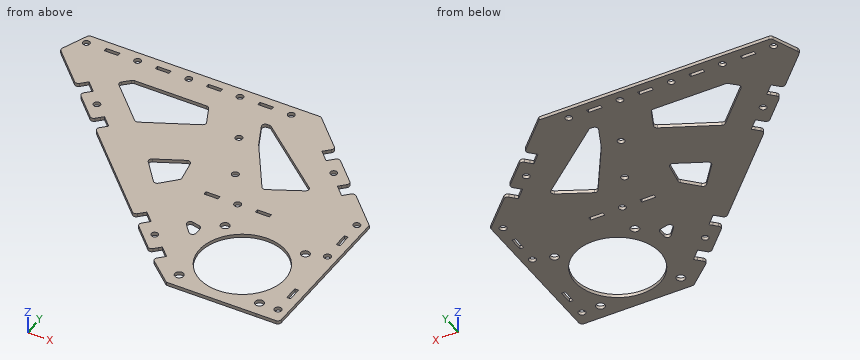
from build123d import *

# Parameters (mm, degrees)
SKETCH_1_R      = 2
SKETCH_1_R_2    = 25
SKETCH_1_R_3    = 2.05
SKETCH_1_R_4    = 2.55
SKETCH_1_W      = 8.1
SKETCH_1_H      = 2.1
SKETCH_1_W_2    = 8.2
SKETCH_1_W_3    = 2.2
SKETCH_1_H_2    = 8.2
EXTRUDE_1_DEPTH = 2
FILLET_2_R      = 2


with BuildPart() as part:
    # 草图1 → 凸台-拉伸1 (new body)
    with BuildSketch(Plane.XY):
        Polygon((7.027428163, -4.999036262), (20.810808237, -16.956988843), (73.227648339, -16.964389058), (87.027428163, -16.964389058), (87.027428163, 75.054738201), (67.497807203, 94.584359161), (63.997628636, 91.084180595), (62.512704395, 89.599256354), (56.785139468, 95.326821282), (58.270063708, 96.811745522), (61.771734574, 100.31043179), (54.027428163, 108.054738201), (46.284614051, 115.797552313), (42.784435485, 112.297373746), (41.299511244, 110.812449505), (35.571946316, 116.540014433), (37.056870557, 118.024938674), (40.557049124, 121.52511724), (21.027428163, 141.054738201), (-114.884210676, 141.054738201), (-121.955278488, 123.983670389), (-100.755816342, 102.784208243), (-97.257364322, 106.282660262), (-95.772440082, 107.767584503), (-90.044875154, 102.040019575), (-91.529799395, 100.555095335), (-95.028251414, 97.056643315), (-87.28543216, 89.313824061), (-79.542612906, 81.571004807), (-76.044160887, 85.069456827), (-74.559236646, 86.554381067), (-68.831671719, 80.82681614), (-70.316595959, 79.341891899), (-73.815047978, 75.84343988), (-21.559856849, 23.58824875), (-18.061404829, 27.086700769), (-16.576480589, 28.57162501), (-10.848915661, 22.844060082), (-12.333839902, 21.359135842), (-15.832291921, 17.860683822), (-8.089472667, 10.117864568), (-0.346653413, 2.375045314), (3.151798606, 5.873497334), (4.636722847, 7.358421574), (10.364287774, 1.630856647), (8.879363534, 0.145932406), (5.380911515, -3.352519613), align=None)
        with Locations((-52.972571837, 135.054738201)):
            Circle(SKETCH_1_R, mode=Mode.SUBTRACT)
        with Locations((47.027428163, 15.054738201)):
            Circle(SKETCH_1_R_2, mode=Mode.SUBTRACT)
        with Locations(Location((-22.972571837, 135.054738201, 0), (0, 0, 180))):
            Circle(SKETCH_1_R, mode=Mode.SUBTRACT)
        with Locations((7.027428163, 135.054738201)):
            Circle(SKETCH_1_R, mode=Mode.SUBTRACT)
        with Locations(Location((-112.972571837, 135.054738201, 0), (0, 0, 180))):
            Circle(SKETCH_1_R, mode=Mode.SUBTRACT)
        with Locations((-82.972571837, 135.054738201)):
            Circle(SKETCH_1_R, mode=Mode.SUBTRACT)
        with Locations((49.784787476, 103.812097514)):
            Circle(SKETCH_1_R, mode=Mode.SUBTRACT)
        with Locations((-83.04451802, 93.554738201)):
            Circle(SKETCH_1_R, mode=Mode.SUBTRACT)
        with Locations((20.275835807, 57.054738201)):
            Circle(SKETCH_1_R_3, mode=Mode.SUBTRACT)
        with Locations((70.527428163, -8.445261799)):
            Circle(SKETCH_1_R_4, mode=Mode.SUBTRACT)
        with Locations((23.527428163, -8.445261799)):
            Circle(SKETCH_1_R_4, mode=Mode.SUBTRACT)
        with Locations((23.527428163, 38.554738201)):
            Circle(SKETCH_1_R_4, mode=Mode.SUBTRACT)
        with Locations((70.527428163, 38.554738201)):
            Circle(SKETCH_1_R_4, mode=Mode.SUBTRACT)
        with Locations((81.392055944, 72.204829046)):
            Circle(SKETCH_1_R_3, mode=Mode.SUBTRACT)
        with Locations((81.392055944, -8.445261799)):
            Circle(SKETCH_1_R_3, mode=Mode.SUBTRACT)
        with Locations((81.392055944, 42.204829046)):
            Circle(SKETCH_1_R_3, mode=Mode.SUBTRACT)
        with Locations((6.845259268, 78.140743367)):
            Circle(SKETCH_1_R_3, mode=Mode.SUBTRACT)
        with Locations(Location((-3.848558527, 14.358778708, 0), (0, 0, 180))):
            Circle(SKETCH_1_R, mode=Mode.SUBTRACT)
        with Locations((-6.58531727, 105.226748532)):
            Circle(SKETCH_1_R_3, mode=Mode.SUBTRACT)
        with Locations((-37.972571837, 135.054738201)):
            Rectangle(SKETCH_1_W, SKETCH_1_H, mode=Mode.SUBTRACT)
        with Locations((-7.972571837, 135.054738201)):
            Rectangle(SKETCH_1_W, SKETCH_1_H, mode=Mode.SUBTRACT)
        with Locations((-97.972571837, 135.054738201)):
            Rectangle(SKETCH_1_W, SKETCH_1_H, mode=Mode.SUBTRACT)
        with Locations((-67.972571837, 135.054738201)):
            Rectangle(SKETCH_1_W, SKETCH_1_H, mode=Mode.SUBTRACT)
        with Locations((5.275835807, 57.054738201)):
            Rectangle(SKETCH_1_W_2, SKETCH_1_H, mode=Mode.SUBTRACT)
        with Locations((35.275835807, 57.054738201)):
            Rectangle(SKETCH_1_W_2, SKETCH_1_H, mode=Mode.SUBTRACT)
        Polygon((-26.317798475, 106.3059132), (-58.783300448, 90.506724064), (-82.786741677, 114.510165293), (-76.96930946, 120.054738201), (-32.606331473, 120.054738201), align=None, mode=Mode.SUBTRACT)
        Polygon((47.299709176, 85.219712632), (24.92619293, 73.952191934), (4.862626833, 105.451990707), (-2.731253041, 122.054738201), (2.37892986, 122.054738201), align=None, mode=Mode.SUBTRACT)
        Polygon((-14.950211349, 60.939664471), (-17.845757969, 77.065019133), (-38.30861977, 67.106860342), (-24.982934729, 50.626518371), align=None, mode=Mode.SUBTRACT)
        Polygon((2.01437662, 34.262984309), (13.802642778, 20.368597473), (13.802642778, 31.594822975), align=None, mode=Mode.SUBTRACT)
        with Locations((81.392055944, 57.204829046)):
            Rectangle(SKETCH_1_W_3, SKETCH_1_H_2, mode=Mode.SUBTRACT)
        with Locations((81.392055944, 6.554738201)):
            Rectangle(SKETCH_1_W_3, SKETCH_1_H_2, mode=Mode.SUBTRACT)
    extrude(amount=EXTRUDE_1_DEPTH)

    # 圆角2
    fillet_2_edges = [part.edges().sort_by_distance(p)[0] for p in [
        (-26.317798475, 106.3059132, 1),
        (-32.606331473, 120.054738201, 1),
        (-76.96930946, 120.054738201, 1),
        (-82.786741677, 114.510165293, 1),
        (-58.783300448, 90.506724064, 1),
        (47.299709176, 85.219712632, 1),
        (2.37892986, 122.054738201, 1),
        (-2.731253041, 122.054738201, 1),
        (24.92619293, 73.952191934, 1),
        (-24.982934729, 50.626518371, 1),
        (-14.950211349, 60.939664471, 1),
        (-17.845757969, 77.065019133, 1),
        (-38.30861977, 67.106860342, 1),
        (13.802642778, 31.594822975, 1),
        (2.01437662, 34.262984309, 1),
        (13.802642778, 20.368597473, 1),
        (40.557049124, 121.52511724, 1),
        (46.284614051, 115.797552313, 1),
        (61.771734574, 100.31043179, 1),
        (67.497807203, 94.584359161, 1),
        (87.027428163, -16.964389058, 1),
        (5.380911515, -3.352519613, 1),
        (-0.346653413, 2.375045314, 1),
        (-15.832291921, 17.860683822, 1),
        (-21.559856849, 23.58824875, 1),
        (-73.815047978, 75.84343988, 1),
        (-79.542612906, 81.571004807, 1),
        (-95.028251414, 97.056643315, 1),
        (-100.755816342, 102.784208243, 1),
        (-121.955278488, 123.983670389, 1),
        (-114.884210676, 141.054738201, 1),
    ]]
    fillet(fillet_2_edges, radius=FILLET_2_R)


solid = part.part
Input: part model. Units: mm. Frame: model coordinates. Round coordinates to 2 decimals unless told otherwise and drop trailing zeros. Order: outer loops, then holes, each group sorted by start corner. A loop starts at its lowest first (then second) coordinate and runs counter-clockwise, first axis right, second up.
1. Material intervals for line 1 (X direction, y = 71, z = 1); line 2 (Y direction, x = 48, z = 0.7); line 3 (Y direction, x = -35, z = 1.25), sorted ascending.
The answers:
line 1: x = -68.97 to -30.31, -16.76 to 79.73, 83.05 to 87.03
line 2: y = -16.96 to -9.93, 40.04 to 102.91, 104.71 to 114.08
line 3: y = 37.03 to 63.01, 68.72 to 102.08, 120.05 to 134, 136.1 to 141.05
2. Cut plane B-B, the plane z = 0.65. State how many separate pieces and enclosed holes the cut face has, then the cut area to 3 significant figures.
The answers:
separate pieces: 1
enclosed holes: 31
area: 15,900 mm2
3. Cut plane A-A, the plane x = -47.5. Output: boundary loops of the cut face in (y, z), then the cut area to 3 significant figures.
The answers:
outline: (49.53, 0) - (96, 0) - (96, 2) - (49.53, 2) - close; (120.05, 0) - (141.05, 0) - (141.05, 2) - (120.05, 2) - close
area: 135 mm2
4. Pin query (flat end, axial travel): P1, Ø5.5, axis at x = 81.39, y = -8.45, coming from the +Z side; P2, Ø3.5, axis at x = 81.39, y = 42.2, coming from the +Z side; P3, Ø0.6, axis at y = 7, z = 0.5, coming from the -X side; P4, Ø0.6, axis at x = -38, z = 1, coming from the -Y side. Return the tip coordinate at first contact, or that it passes through.
The answers:
P1: stops at z = 2
P2: passes through
P3: stops at x = -5.27
P4: stops at y = 39.73
